Input: part model. Units: mm. Frame: model coordinates. A direction names the side the tool comes from. Round coordinates to 2 decimals unless told otherwise and drop trailing zeros. Loops run counter-clockwise (first coordinate to the right, second up) from the corner with the lowest first, then second, coordinate; pieces in that order, holes last. Notation, with made-up numbers: (-6.75, 2) - (5.25, 2) arc R30 ccw to (5.25, 38) - close; hole circle Ø1 at (-22, 34.5). An arc over 180 degrees is marked (long way). Use CSV: the item, a comma, the result in double quotes. Start each with the question number.
1. Pin query (flat end, axial travel): P1, Ø1.3, axis at x = -12.5, y = -3.5, coming from the -Z side; P2, Ø1, axis at x = -0.5, z = 45.5, coming from the -Y side; P3, Ø12, axis at y = -8.5, z = 2, coming from the +X side. Return the tip coordinate at first contact, or that it passes through.
2. Pull-direction query (X, two-part tool) for faces 4 (the cylindrical face through (-2.005, -2.969, 97.088)), 5 (the flat face through (-18, -31, 96.305)), 6 (the flat face through (-12, -3, -7.598)); classes: +X half, -X half, draft (parallel to the pull), parting line (faces both ways), or undercut.
3. Material intervals for probe 1 along X at (y, z) = (16, 39); probe 2 along X at (y, z) = (0, 44.5); probe 3 along Z at (x, y) = (-3.5, 21.5), sorted ascending. Write a range as from..to.
4. Cut plane D-D (y = 10.5). Return loops of the section in (x, z).
5. Access query for faces 1 (the cylindrical face through (-12.622, -2.229, 96.524)), 2 (the cylindrical face through (-0.796, 6.911, 54.144)), 3 (the flat face through (-19, -31, 96.013)). Directions: +Z, -Z, +X, -X, +Y, -Y. A direction counts if a zero-diameter tool reaches every point of the face in a straight line with its end or side. Return the directions, or none.
6. Cut plane A-A (y = -6). Return loops of the section in (x, z).
7. Cut plane C-C (x = -2.5). Return loops of the section in (y, z).
8. Cut plane B-B (z = 60). Return loops of the section in (x, y).
```python
from build123d import *

# Parameters (mm, degrees)
SKETCH1_W           = 107.95
SKETCH1_H           = 60.325
BOSS_EXTRUDE1_DEPTH = 19.05
FILLET1_R           = 2.54
SKETCH5_R           = 1.27
CUT_EXTRUDE2_DEPTH  = 2.54
CUT_EXTRUDE3_START  = -2.54
SKETCH6_R           = 1.27
CUT_EXTRUDE3_DEPTH  = 2.54
BOSS_EXTRUDE3_DEPTH = 0.9017
SKETCH8_R           = 1.016
BOSS_EXTRUDE4_DEPTH = 3.048
SKETCH9_W           = 7.9375
SKETCH9_H           = 4.064
CUT_EXTRUDE4_DEPTH  = 4.064
BOSS_EXTRUDE5_DEPTH = 5.334


with BuildPart() as part:
    # Sketch1 → Boss-Extrude1 (new body)
    with BuildSketch(Plane(origin=(-20.290873615, 0, 0), x_dir=(0, 0, -1), z_dir=(1, 0, 0))):
        with Locations((-43.836998095, -3.355404983)):
            Rectangle(SKETCH1_W, SKETCH1_H)
    extrude(amount=BOSS_EXTRUDE1_DEPTH)

    # Fillet1
    fillet1_edges = [part.edges().sort_by_distance(p)[0] for p in [
        (-1.240873615, -3.355404983, -10.138001905),
        (-1.240873615, 26.807095017, 43.836998095),
        (-1.240873615, -3.355404983, 97.811998095),
        (-1.240873615, -33.517904983, 43.836998095),
        (-10.765873615, 26.807095017, 97.811998095),
        (-10.765873615, 26.807095017, -10.138001905),
        (-10.765873615, -33.517904983, -10.138001905),
        (-10.765873615, -33.517904983, 97.811998095),
    ]]
    fillet(fillet1_edges, radius=FILLET1_R)

    # Sketch5 → Cut-Extrude2 (cut)
    with BuildSketch(Plane(origin=(0, 0, -10.138001905), x_dir=(-1, 0, 0), z_dir=(0, 0, -1))):
        with Locations((12.035873615, -3.355404983)):
            Circle(SKETCH5_R)
    extrude(amount=-CUT_EXTRUDE2_DEPTH, mode=Mode.SUBTRACT)

    # Sketch6 → Cut-Extrude3 (cut)
    with BuildSketch(Plane.XY.offset(97.811998095).offset(CUT_EXTRUDE3_START)):
        with Locations(Location((-12.035873615, -3.355404983, 0), (0, 0, 180))):
            Circle(SKETCH6_R)
    extrude(amount=CUT_EXTRUDE3_DEPTH, mode=Mode.SUBTRACT)

    # Sketch7 → Boss-Extrude3 (add)
    with BuildSketch(Plane(origin=(-1.240873615, 0, 0), x_dir=(0, 0, -1), z_dir=(1, 0, 0))):
        with BuildLine():
            Line((-52.328218095, 7.674545017), (-35.345778095, 7.674545017))
            ThreePointArc((-35.345778095, 7.674545017), (-33.549726871, 6.930596241), (-32.805778095, 5.134545017))
            Line((-32.805778095, 5.134545017), (-32.805778095, -11.845354983))
            ThreePointArc((-32.805778095, -11.845354983), (-33.549726871, -13.641406207), (-35.345778095, -14.385354983))
            Line((-35.345778095, -14.385354983), (-52.328218095, -14.385354983))
            ThreePointArc((-52.328218095, -14.385354983), (-54.124269319, -13.641406207), (-54.868218095, -11.845354983))
            Line((-54.868218095, -11.845354983), (-54.868218095, 5.134545017))
            ThreePointArc((-54.868218095, 5.134545017), (-54.124269319, 6.930596241), (-52.328218095, 7.674545017))
        make_face()
    extrude(amount=BOSS_EXTRUDE3_DEPTH)

    # Sketch8 → Boss-Extrude4 (add)
    with BuildSketch(Plane.ZY.offset(20.290873615)):
        with Locations(Location((88.540998095, 21.281395003, 0), (0, 0, 180))):
            Circle(SKETCH8_R)
    extrude(amount=BOSS_EXTRUDE4_DEPTH)

    # Sketch9 → Cut-Extrude4 (cut)
    with BuildSketch(Plane.ZY.offset(20.290873615)):
        with Locations((92.336317085, -30.791056829)):
            Rectangle(SKETCH9_W, SKETCH9_H)
    extrude(amount=-CUT_EXTRUDE4_DEPTH, mode=Mode.SUBTRACT)

    # Sketch10 → Boss-Extrude5 (add)
    with BuildSketch(Plane.ZY.offset(16.226873615)):
        Polygon((88.868929932, -28.90840101), (88.868929932, -32.323313533), (95.680387965, -32.323313533), (95.680387965, -28.90840101), (96.013379651, -28.90840101), (96.013379651, -32.648312217), (88.518168835, -32.648312217), (88.518168835, -28.90840101), align=None)
    extrude(amount=BOSS_EXTRUDE5_DEPTH)


solid = part.part
```
Established:
1,P1,"stops at z = -7.6"
1,P2,"stops at y = -14.39"
1,P3,"stops at x = -1.24"
2,face 4,"+X half"
2,face 5,"draft"
2,face 6,"undercut"
3,probe 1,"x = -20.29..-1.24"
3,probe 2,"x = -20.29..-0.34"
3,probe 3,"z = -10.12..97.8"
4,outline,"(-20.29, -10.14) - (-3.78, -10.14) arc R2.54 ccw to (-1.24, -7.6) - (-1.24, 95.27) arc R2.54 ccw to (-3.78, 97.81) - (-20.29, 97.81) - close"
5,face 1,"+Z"
5,face 2,"+Z, +X, +Y"
5,face 3,"-X"
6,outline,"(-20.29, -10.14) - (-3.78, -10.14) arc R2.54 ccw to (-1.24, -7.6) - (-1.24, 32.81) - (-0.34, 32.81) - (-0.34, 54.87) - (-1.24, 54.87) - (-1.24, 95.27) arc R2.54 ccw to (-3.78, 97.81) - (-20.29, 97.81) - close"
7,outline,"(-33.17, -7.6) arc R2.19 ccw to (-30.98, -9.79) - (24.27, -9.79) arc R2.19 ccw to (26.46, -7.6) - (26.46, 95.27) arc R2.19 ccw to (24.27, 97.47) - (-30.98, 97.47) arc R2.19 ccw to (-33.17, 95.27) - close"
8,outline,"(-20.29, -33.52) - (-3.78, -33.52) arc R2.54 ccw to (-1.24, -30.98) - (-1.24, 24.27) arc R2.54 ccw to (-3.78, 26.81) - (-20.29, 26.81) - close"
